from build123d import *

# Parameters (mm, degrees)
CROQUIS1_R              = 1.55
CROQUIS1_R_2            = 4
SALIENTE_EXTRUIR1_DEPTH = 120
CORTAR_EXTRUIR1_DEPTH   = 117
CORTAR_EXTRUIR2_REACH   = 129.299
CROQUIS3_R              = 1.55
MATRIZC1_COUNT          = 8


with BuildPart() as part:
    # Croquis1 → Saliente-Extruir1 (new body)
    with BuildSketch(Plane(origin=(0, 0, 0), x_dir=(1, 0, 0), z_dir=(0, 1, 0))):
        Polygon((19, -7.870057685), (19, 7.870057685), (7.870057685, 19), (-7.870057685, 19), (-19, 7.870057685), (-19, -7.870057685), (-7.870057685, -19), (7.870057685, -19), align=None)
        with Locations(Location((0, 11, 0), (0, 0, 270))):
            Circle(CROQUIS1_R, mode=Mode.SUBTRACT)
        with Locations(Location((0, 0, 0), (0, 0, 270))):
            Circle(CROQUIS1_R_2, mode=Mode.SUBTRACT)
        with Locations(Location((7.778174593, 7.778174593, 0), (0, 0, 270))):
            Circle(CROQUIS1_R, mode=Mode.SUBTRACT)
        with Locations(Location((11, 0, 0), (0, 0, 270))):
            Circle(CROQUIS1_R, mode=Mode.SUBTRACT)
        with Locations(Location((7.778174593, -7.778174593, 0), (0, 0, 270))):
            Circle(CROQUIS1_R, mode=Mode.SUBTRACT)
        with Locations(Location((0, -11, 0), (0, 0, 270))):
            Circle(CROQUIS1_R, mode=Mode.SUBTRACT)
        with Locations(Location((-7.778174593, -7.778174593, 0), (0, 0, 270))):
            Circle(CROQUIS1_R, mode=Mode.SUBTRACT)
        with Locations(Location((-11, 0, 0), (0, 0, 270))):
            Circle(CROQUIS1_R, mode=Mode.SUBTRACT)
        with Locations(Location((-7.778174593, 7.778174593, 0), (0, 0, 270))):
            Circle(CROQUIS1_R, mode=Mode.SUBTRACT)
    extrude(amount=SALIENTE_EXTRUIR1_DEPTH)

    # Croquis2 → Cortar-Extruir1 (cut)
    with BuildSketch(Plane(origin=(0, 120, 0), x_dir=(1, 0, 0), z_dir=(0, 1, 0))):
        Polygon((7.04163056, 17), (-7.04163056, 17), (-17, 7.04163056), (-17, -7.04163056), (-7.04163056, -17), (7.04163056, -17), (17, -7.04163056), (17, 7.04163056), align=None)
    extrude(amount=-CORTAR_EXTRUIR1_DEPTH, mode=Mode.SUBTRACT)

    # Croquis3 → Cortar-Extruir2 (cut, up to next)
    with BuildSketch(Plane(origin=(0, 0, -19), x_dir=(-1, 0, 0), z_dir=(0, 0, -1)), mode=Mode.PRIVATE) as cortar_extruir2_sk1:
        with Locations((0, 115)):
            Circle(CROQUIS3_R)
    cortar_extruir2_tool1 = extrude(cortar_extruir2_sk1.sketch, amount=-CORTAR_EXTRUIR2_REACH, mode=Mode.PRIVATE) & part.part
    # Croquis3 → Cortar-Extruir2 (cut, up to next)
    with BuildSketch(Plane(origin=(0, 0, -19), x_dir=(-1, 0, 0), z_dir=(0, 0, -1)), mode=Mode.PRIVATE) as cortar_extruir2_sk2:
        with Locations((0, 105)):
            Circle(CROQUIS3_R)
    cortar_extruir2_tool2 = extrude(cortar_extruir2_sk2.sketch, amount=-CORTAR_EXTRUIR2_REACH, mode=Mode.PRIVATE) & part.part
    # Croquis3 → Cortar-Extruir2 (cut, up to next)
    with BuildSketch(Plane(origin=(0, 0, -19), x_dir=(-1, 0, 0), z_dir=(0, 0, -1)), mode=Mode.PRIVATE) as cortar_extruir2_sk3:
        with Locations((0, 95)):
            Circle(CROQUIS3_R)
    cortar_extruir2_tool3 = extrude(cortar_extruir2_sk3.sketch, amount=-CORTAR_EXTRUIR2_REACH, mode=Mode.PRIVATE) & part.part
    # Croquis3 → Cortar-Extruir2 (cut, up to next)
    with BuildSketch(Plane(origin=(0, 0, -19), x_dir=(-1, 0, 0), z_dir=(0, 0, -1)), mode=Mode.PRIVATE) as cortar_extruir2_sk4:
        with Locations((0, 85)):
            Circle(CROQUIS3_R)
    cortar_extruir2_tool4 = extrude(cortar_extruir2_sk4.sketch, amount=-CORTAR_EXTRUIR2_REACH, mode=Mode.PRIVATE) & part.part
    # Croquis3 → Cortar-Extruir2 (cut, up to next)
    with BuildSketch(Plane(origin=(0, 0, -19), x_dir=(-1, 0, 0), z_dir=(0, 0, -1)), mode=Mode.PRIVATE) as cortar_extruir2_sk5:
        with Locations((0, 75)):
            Circle(CROQUIS3_R)
    cortar_extruir2_tool5 = extrude(cortar_extruir2_sk5.sketch, amount=-CORTAR_EXTRUIR2_REACH, mode=Mode.PRIVATE) & part.part
    # Croquis3 → Cortar-Extruir2 (cut, up to next)
    with BuildSketch(Plane(origin=(0, 0, -19), x_dir=(-1, 0, 0), z_dir=(0, 0, -1)), mode=Mode.PRIVATE) as cortar_extruir2_sk6:
        with Locations((0, 65)):
            Circle(CROQUIS3_R)
    cortar_extruir2_tool6 = extrude(cortar_extruir2_sk6.sketch, amount=-CORTAR_EXTRUIR2_REACH, mode=Mode.PRIVATE) & part.part
    # Croquis3 → Cortar-Extruir2 (cut, up to next)
    with BuildSketch(Plane(origin=(0, 0, -19), x_dir=(-1, 0, 0), z_dir=(0, 0, -1)), mode=Mode.PRIVATE) as cortar_extruir2_sk7:
        with Locations((0, 55)):
            Circle(CROQUIS3_R)
    cortar_extruir2_tool7 = extrude(cortar_extruir2_sk7.sketch, amount=-CORTAR_EXTRUIR2_REACH, mode=Mode.PRIVATE) & part.part
    # Croquis3 → Cortar-Extruir2 (cut, up to next)
    with BuildSketch(Plane(origin=(0, 0, -19), x_dir=(-1, 0, 0), z_dir=(0, 0, -1)), mode=Mode.PRIVATE) as cortar_extruir2_sk8:
        with Locations((0, 45)):
            Circle(CROQUIS3_R)
    cortar_extruir2_tool8 = extrude(cortar_extruir2_sk8.sketch, amount=-CORTAR_EXTRUIR2_REACH, mode=Mode.PRIVATE) & part.part
    # Croquis3 → Cortar-Extruir2 (cut, up to next)
    with BuildSketch(Plane(origin=(0, 0, -19), x_dir=(-1, 0, 0), z_dir=(0, 0, -1)), mode=Mode.PRIVATE) as cortar_extruir2_sk9:
        with Locations((0, 35)):
            Circle(CROQUIS3_R)
    cortar_extruir2_tool9 = extrude(cortar_extruir2_sk9.sketch, amount=-CORTAR_EXTRUIR2_REACH, mode=Mode.PRIVATE) & part.part
    # Croquis3 → Cortar-Extruir2 (cut, up to next)
    with BuildSketch(Plane(origin=(0, 0, -19), x_dir=(-1, 0, 0), z_dir=(0, 0, -1)), mode=Mode.PRIVATE) as cortar_extruir2_sk10:
        with Locations((0, 25)):
            Circle(CROQUIS3_R)
    cortar_extruir2_tool10 = extrude(cortar_extruir2_sk10.sketch, amount=-CORTAR_EXTRUIR2_REACH, mode=Mode.PRIVATE) & part.part
    cortar_extruir2_1 = cortar_extruir2_tool1.solids().sort_by_distance((0, 115, -19))[0]
    add(cortar_extruir2_1, mode=Mode.SUBTRACT)
    cortar_extruir2_2 = cortar_extruir2_tool2.solids().sort_by_distance((0, 105, -19))[0]
    add(cortar_extruir2_2, mode=Mode.SUBTRACT)
    cortar_extruir2_3 = cortar_extruir2_tool3.solids().sort_by_distance((0, 95, -19))[0]
    add(cortar_extruir2_3, mode=Mode.SUBTRACT)
    cortar_extruir2_4 = cortar_extruir2_tool4.solids().sort_by_distance((0, 85, -19))[0]
    add(cortar_extruir2_4, mode=Mode.SUBTRACT)
    cortar_extruir2_5 = cortar_extruir2_tool5.solids().sort_by_distance((0, 75, -19))[0]
    add(cortar_extruir2_5, mode=Mode.SUBTRACT)
    cortar_extruir2_6 = cortar_extruir2_tool6.solids().sort_by_distance((0, 65, -19))[0]
    add(cortar_extruir2_6, mode=Mode.SUBTRACT)
    cortar_extruir2_7 = cortar_extruir2_tool7.solids().sort_by_distance((0, 55, -19))[0]
    add(cortar_extruir2_7, mode=Mode.SUBTRACT)
    cortar_extruir2_8 = cortar_extruir2_tool8.solids().sort_by_distance((0, 45, -19))[0]
    add(cortar_extruir2_8, mode=Mode.SUBTRACT)
    cortar_extruir2_9 = cortar_extruir2_tool9.solids().sort_by_distance((0, 35, -19))[0]
    add(cortar_extruir2_9, mode=Mode.SUBTRACT)
    cortar_extruir2_10 = cortar_extruir2_tool10.solids().sort_by_distance((0, 25, -19))[0]
    add(cortar_extruir2_10, mode=Mode.SUBTRACT)
    cortar_extruir2 = cortar_extruir2_1 + cortar_extruir2_2 + cortar_extruir2_3 + cortar_extruir2_4 + cortar_extruir2_5 + cortar_extruir2_6 + cortar_extruir2_7 + cortar_extruir2_8 + cortar_extruir2_9 + cortar_extruir2_10  # Cortar-Extruir2 as one shape, for the pattern or mirror that repeats it

    # MatrizC1: Cortar-Extruir2 ×8 about axis
    matrizc1_axis = Axis((0, 3, 0), (0, 1, 0))
    for i in range(1, MATRIZC1_COUNT):
        add(cortar_extruir2.rotate(matrizc1_axis, i * 360 / MATRIZC1_COUNT), mode=Mode.SUBTRACT)


solid = part.part
Can you work these out from the model? Positions are in its coordinate system, mm. A direction names the side the tool comes from. Give positions to 0.01 mm unless a question says otherwise; leave off trailing zeros. Loops run counter-clockwise (first coordinate to the right, second up) from the corner with the lowest first, then second, coordinate; pieces in that order, holes last. Notation, with made-up numbers: (56, 9.5) - (62, 9.5) arc R19 ccw to (62, 34.5) - close; hole circle Ø11 at (-11.75, -22.5). An arc over 180 degrees is marked (long way). One line per item, written item: value.
(1) If we section it at B-B, the plane x = 0: State how many separate pieces and enclosed holes the cut face has, plus the area to 3 significant figures.
Verdict:
separate pieces: 24
enclosed holes: 0
area: 415 mm^2
(2) I need wall thicknesses on line 1 along X through (y, z) = (1, 0); line 2 along X through (y, z) = (76, -5.5). Which ranges of each line are inside material? Lowest first, please.
Verdict:
line 1: -19 to -12.55, -9.45 to -4, 4 to 9.45, 12.55 to 19
line 2: -19 to -17, 17 to 19
(3) I'm going to push a flat-ended pin straight in: pin 1 (3.5 mm diameter, centred on x = 0, z = -11, fed in from +Y). Where does the tip first touch, or does it pass through?
Verdict:
pin 1: y = 3
(4) If we mould it in two halves opening along X, with no side actions, what happens to faces 1 (the face through (-18.014, 76.537, -0.202)), 2 (the face through (19, 59, 0)), 3 (the face through (12.595, 56.537, 12.881))? For each: released by +X, released by -X, zero draft, split by the parting line, or undercut.
Verdict:
face 1: zero draft
face 2: released by +X
face 3: undercut
(5) If we section it at A-A, the plane y = 88: List the corners of the cut face in (x, z) for me, plus the area to 3 significant figures.
Verdict:
outline: (-19, -7.87) - (-7.87, -19) - (7.87, -19) - (19, -7.87) - (19, 7.87) - (7.87, 19) - (-7.87, 19) - (-19, 7.87) - close; hole (-17, -7.04) - (-7.04, -17) - (7.04, -17) - (17, -7.04) - (17, 7.04) - (7.04, 17) - (-7.04, 17) - (-17, 7.04) - close
area: 239 mm^2
(6) On a 3-axis mill with a long thin cutter (end or side, diameter ignored), from which of +Z, -Z, +X, -X, +Y, -Y can I reach the whole of each face in a straight line? I mean faces 4 (the face through (-12.975, 103.487, 12.5)), 5 (the face through (12.09, 62.32, -11.95)). Say none if no direction works.
Verdict:
face 4: none
face 5: +Y
